Source: CAD feature listing. Evaluate the final solid. Frame: model axes, mm. Round coordinates to 2 decimals unless told otherwise and drop trailing zeros. Write each loop counter-clockwise with the first axis right and the second up, starting at its lowest first coordinate (ties: lowest second). Pieces come first, ordered by that corner, then holes. Notation, with made-up numbers: M 59,58 L 118,58 A25 ccw 118,96 Z; hole C -1,18 d10. An arc over 180 degrees is marked long. Use a Markdown table: item, result.
```python
from build123d import *

# Parameters (mm, degrees)
BOSS_EXTRUDE1_DEPTH = 3.175
SKETCH3_W           = 3.175
SKETCH3_H           = 31.75
SKETCH3_H_2         = 29.028571429
CUT_EXTRUDE1_DEPTH  = 416.694688143
SKETCH4_R           = 1.5
CUT_EXTRUDE2_DEPTH  = 3.175
SKETCH5_W           = 3.175
SKETCH5_H           = 44.45
SKETCH5_W_2         = 59.103846153
SKETCH5_H_2         = 6.35
SKETCH5_W_3         = 59.103846154
CUT_EXTRUDE3_DEPTH  = 3.175


with BuildPart() as part:
    # Sketch1 → Boss-Extrude1 (new body)
    with BuildSketch(Plane(origin=(0, 0, 0), x_dir=(0, 0, -1), z_dir=(1, 0, 0))):
        Polygon((-384.175, 152.4), (-384.175, 107.95), (-381, 107.95), (-381, 63.5), (-384.175, 63.5), (-384.175, 19.05), (-381, 19.05), (-381, -25.4), (-384.175, -25.4), (-384.175, -69.85), (-381, -69.85), (-381, -114.3), (-384.175, -114.3), (-384.175, -152.4), (-325.071153846, -152.4), (-325.071153846, -158.75), (-265.967307692, -158.75), (-265.967307692, -152.4), (-206.863461538, -152.4), (-206.863461538, -158.75), (-147.759615385, -158.75), (-147.759615385, -152.4), (-88.655769231, -152.4), (-88.655769231, -158.75), (-29.551923077, -158.75), (-29.551923077, -152.4), (29.551923077, -152.4), (29.551923077, -158.75), (88.655769231, -158.75), (88.655769231, -152.4), (147.759615385, -152.4), (147.759615385, -158.75), (206.863461538, -158.75), (206.863461538, -152.4), (265.967307692, -152.4), (265.967307692, -158.75), (325.071153846, -158.75), (325.071153846, -152.4), (384.175, -152.4), (384.175, -114.3), (381, -114.3), (381, -69.85), (384.175, -69.85), (384.175, -25.4), (381, -25.4), (381, 19.05), (384.175, 19.05), (384.175, 63.5), (381, 63.5), (381, 107.95), (384.175, 107.95), (384.175, 152.4), align=None)
    extrude(amount=BOSS_EXTRUDE1_DEPTH)

    # Sketch3 → Cut-Extrude1 (cut, through all)
    with BuildSketch(Plane(origin=(3.175, 0, 0), x_dir=(0, 0, -1), z_dir=(1, 0, 0))):
        with Locations((-123.823769685, -104.775)):
            Rectangle(SKETCH3_W, SKETCH3_H)
        with Locations((-123.823769685, -41.275)):
            Rectangle(SKETCH3_W, SKETCH3_H)
        with Locations((-123.823769685, 22.225)):
            Rectangle(SKETCH3_W, SKETCH3_H)
        with Locations((-123.823769685, 85.725)):
            Rectangle(SKETCH3_W, SKETCH3_H)
        with Locations((-130.176230315, 61.685714285)):
            Rectangle(SKETCH3_W, SKETCH3_H_2)
        with Locations((-130.176230315, 3.628571428)):
            Rectangle(SKETCH3_W, SKETCH3_H_2)
        with Locations((-130.176230315, -54.428571428)):
            Rectangle(SKETCH3_W, SKETCH3_H_2)
        with Locations((-130.176230315, -112.485714286)):
            Rectangle(SKETCH3_W, SKETCH3_H_2)
        with Locations((130.176230315, 85.725)):
            Rectangle(SKETCH3_W, SKETCH3_H)
        with Locations((123.823769685, 61.685714285)):
            Rectangle(SKETCH3_W, SKETCH3_H_2)
        with Locations((130.176230315, 22.225)):
            Rectangle(SKETCH3_W, SKETCH3_H)
        with Locations((123.823769685, 3.628571428)):
            Rectangle(SKETCH3_W, SKETCH3_H_2)
        with Locations((130.176230315, -41.275)):
            Rectangle(SKETCH3_W, SKETCH3_H)
        with Locations((123.823769685, -54.428571428)):
            Rectangle(SKETCH3_W, SKETCH3_H_2)
        with Locations((130.176230315, -104.775)):
            Rectangle(SKETCH3_W, SKETCH3_H)
        with Locations((123.823769685, -112.485714286)):
            Rectangle(SKETCH3_W, SKETCH3_H_2)
    extrude(amount=-CUT_EXTRUDE1_DEPTH, mode=Mode.SUBTRACT)

    # Sketch4 → Cut-Extrude2 (cut)
    with BuildSketch(Plane(origin=(3.175, 0, 0), x_dir=(0, 0, -1), z_dir=(1, 0, 0))):
        with Locations((-365.125, 137.4)):
            Circle(SKETCH4_R)
        with Locations((-365.125, 121.65)):
            Circle(SKETCH4_R)
        with Locations((365.125, 137.4)):
            Circle(SKETCH4_R)
        with Locations((365.125, 121.65)):
            Circle(SKETCH4_R)
    extrude(amount=-CUT_EXTRUDE2_DEPTH, mode=Mode.SUBTRACT)

    # Sketch5 → Cut-Extrude3 (cut)
    with BuildSketch(Plane(origin=(3.175, 0, 0), x_dir=(0, 0, -1), z_dir=(1, 0, 0))):
        with Locations((-382.5875, 41.275)):
            Rectangle(SKETCH5_W, SKETCH5_H)
        with Locations((-382.5875, -47.625)):
            Rectangle(SKETCH5_W, SKETCH5_H)
        with Locations((-177.311538462, -155.575)):
            Rectangle(SKETCH5_W_2, SKETCH5_H_2)
        with Locations((-59.103846154, -155.575)):
            Rectangle(SKETCH5_W_3, SKETCH5_H_2)
        with Locations((59.103846154, -155.575)):
            Rectangle(SKETCH5_W_3, SKETCH5_H_2)
        with Locations((177.311538462, -155.575)):
            Rectangle(SKETCH5_W_2, SKETCH5_H_2)
        with Locations((382.5875, -47.625)):
            Rectangle(SKETCH5_W, SKETCH5_H)
        with Locations((382.5875, 41.275)):
            Rectangle(SKETCH5_W, SKETCH5_H)
    extrude(amount=-CUT_EXTRUDE3_DEPTH, mode=Mode.SUBTRACT)


solid = part.part
```
Q1. Section A-A on y = 58.5. Return loops of the section in (x, z) (3 decimals).
Results are:
| item | result |
|---|---|
| outline | M 0,-381 L 3.175,-381 L 3.175,-125.411 L 0,-125.411 Z; M 0,-122.236 L 3.175,-122.236 L 3.175,128.589 L 0,128.589 Z; M 0,131.764 L 3.175,131.764 L 3.175,381 L 0,381 Z |
Q2. Line query: L1, parallel to Z at x = 2.1, y = 121.65 (3 decimals); L2, parallel to Z at x = 1.4, y = -53.5; L3, parallel to Z at x = 1.95, y = -9.5. Output: solid intervals per line, ascending.
Results are:
| item | result |
|---|---|
| L1 | -384.175 to -366.625, -363.625 to 363.625, 366.625 to 384.175 |
| L2 | -381 to -131.76, -128.59 to -125.41, -122.24 to 122.24, 125.41 to 128.59, 131.76 to 381 |
| L3 | -381 to -125.41, -122.24 to 128.59, 131.76 to 381 |
Q3. Section B-B on x = 2. Give the number of separate pieces and of enclosed holes in the cut face, plus the area to 3 significant figures.
Results are:
| item | result |
|---|---|
| separate pieces | 1 |
| enclosed holes | 20 |
| area | 232,000 mm^2 |
Q4. First-contact query: pin 1 Ø1 at (x, z) = (2.5, -123.5) entering from -Y; pin 2 Ø1 at (x, y) = (1.5, 22) entering from -Z. Flat tips, straight axial feed; report the tip coordinate or a pass-through.
Results are:
| item | result |
|---|---|
| pin 1 | y = -152.4 |
| pin 2 | z = -381 |
Q5. Section C-C on z = 257. Return loops of the section in (x, y) (3 decimals).
Results are:
| item | result |
|---|---|
| outline | M 0,-152.4 L 3.175,-152.4 L 3.175,152.4 L 0,152.4 Z |
